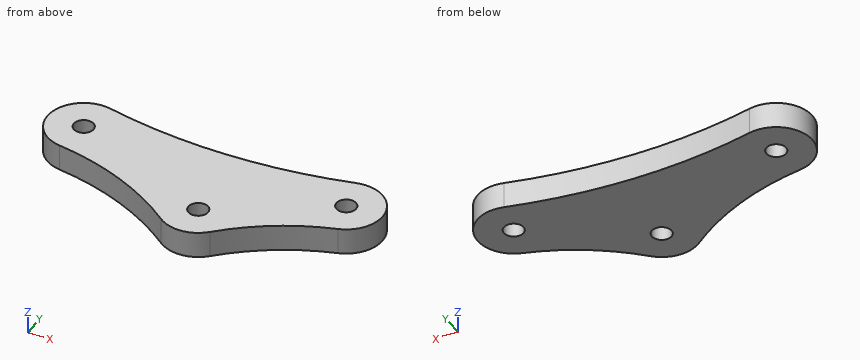
from build123d import *

# Parameters (mm, degrees)
SKETCH1_R           = 1.5
BOSS_EXTRUDE1_DEPTH = 4


with BuildPart() as part:
    # Sketch1 → Boss-Extrude1 (new body)
    with BuildSketch(Plane.XY):
        with BuildLine():
            ThreePointArc((-38.713450292, 5.347409639), (-45.397441252, 1.057179235), (-40.825882635, -5.437638998))
            ThreePointArc((-40.825882635, -5.437638998), (-30.223624193, -8.515546688), (-20.789672108, -14.24982501))
            ThreePointArc((-20.789672108, -14.24982501), (-17.086113442, -15.460299774), (-13.509973062, -13.913426824))
            ThreePointArc((-13.509973062, -13.913426824), (-6.552111329, -8.667968977), (1.482746603, -5.29636314))
            ThreePointArc((1.482746603, -5.29636314), (5.322790438, 1.384883371), (-1.286549708, 5.347409639))
            ThreePointArc((-1.286549708, 5.347409639), (-20, 3.127913483), (-38.713450292, 5.347409639))
        make_face()
        with Locations((-40, 0)):
            Circle(SKETCH1_R, mode=Mode.SUBTRACT)
        Circle(SKETCH1_R, mode=Mode.SUBTRACT)
        with Locations((-17.34, -9.966162752)):
            Circle(SKETCH1_R, mode=Mode.SUBTRACT)
    extrude(amount=BOSS_EXTRUDE1_DEPTH)


solid = part.part
Design review of the part built by this model. Coordinates are the model's own, in mm. Round coordinates to 2 decimals unless told otherwise and drop trailing zeros. Write each loop counter-clockwise with the first axis right and the second up, starting at its lowest first coordinate (ties: lowest second). Pieces come first, ordered by that corner, then holes. Notation, with made-up numbers: (82, -24) - (95, -24) arc R15 cw to (95, -3) - close; hole circle Ø10 at (0, 1.5). An arc over 180 degrees is marked (long way). Return JSON: item names as keys, results as strings. Group by question number.
Item 1: Insertion check: P1, Ø1.5, axis at x = -7, z = 2, coming from the -Y side; P2, Ø1.5, axis at x = -17, y = -10.5, coming from the +Z side; P3, Ø2, axis at x = -9.5, z = 1.5, coming from the -Y side. Each pin has a flat end and moves straight along its axis. Give the tip position at first contact, or say it passes through.
Item 2: We need section C-C on x = 0. Write out the cut boundary in (y, z).
Item 3: We need section A-A on x = -40. Write out the cut boundary in (y, z).
Item 4: We need section B-B on z = 1.15. Write out the cut boundary in (x, y).
Item 5: We need section D-D on y = -2.25. Write out the cut boundary in (x, z).
Item 6: For probe 1 along Y at (x, z) = (-40, 2.1); probe 2 along Y at (x, z) = (-17.34, 2.75); probe 3 along X at (y, z) = (0.25, 2.1), list the stretches that pass through material, from the lowest coordinate up. Write a range as [from, to].
Model answer:
{
 "1": {"P1": "stops at y = -9.39", "P2": "passes through", "P3": "stops at y = -11.31"},
 "2": {"outline": "(-5.75, 0) - (-1.5, 0) - (-1.5, 4) - (-5.75, 4) - close; (1.5, 0) - (5.5, 0) - (5.5, 4) - (1.5, 4) - close"},
 "3": {"outline": "(-5.57, 0) - (-1.5, 0) - (-1.5, 4) - (-5.57, 4) - close; (1.5, 0) - (5.5, 0) - (5.5, 4) - (1.5, 4) - close"},
 "4": {"outline": "(-40.83, -5.44) arc R42 cw to (-20.79, -14.25) arc R5.5 ccw to (-13.51, -13.91) arc R35.13 cw to (1.48, -5.3) arc R5.5 ccw to (-1.29, 5.35) arc R80 cw to (-38.71, 5.35) arc R5.5 ccw (long way) to start; hole circle Ø3 at (-40, 0); hole circle Ø3 at (-17.34, -9.97); hole circle Ø3 at (0, 0)"},
 "5": {"outline": "(-45.02, 0) - (5.02, 0) - (5.02, 4) - (-45.02, 4) - close"},
 "6": {"probe 1": "y = [-5.57, -1.5], [1.5, 5.5]", "probe 2": "y = [-15.47, -11.47], [-8.47, 3.17]", "probe 3": "x = [-45.49, -41.48], [-38.52, -1.48], [1.48, 5.49]"}
}
